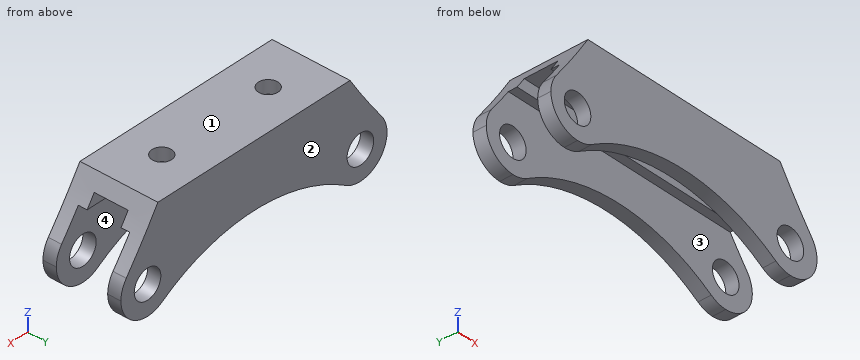
```python
from build123d import *

# Parameters (mm, degrees)
EXTRUDE1_DEPTH            = 47.625
SKETCH4_R                 = 4.7625
SPHERICALHOLES_DEPTH      = 13.7
SPHERICALHOLES_DEPTH_BACK = 13.7
FILLET1_R                 = 9.525
SKETCH5_R                 = 3.175
EXTRUDE2_DEPTH            = 5.318
EXTRUDE3_START            = -47.625
SKETCH6_W                 = 3.81
SKETCH6_H                 = 2.8575
EXTRUDE3_DEPTH            = 95.25
CUT_EXTRUDE1_DEPTH        = 26.4
CUT_EXTRUDE3_DEPTH        = 26.4


with BuildPart() as part:
    # Sketch2 → Extrude1 (new body, symmetric)
    with BuildSketch(Plane(origin=(0, 0, 0), x_dir=(0, 0, -1), z_dir=(1, 0, 0))):
        Polygon((4.318, -8.382), (4.318, 8.382), (31.75, 8.382), (31.75, 12.7), (0, 12.7), (0, -12.7), (31.75, -12.7), (31.75, -8.382), align=None)
    extrude(amount=EXTRUDE1_DEPTH, both=True)

    # Sketch4 → SphericalHoles (cut, two sides)
    with BuildSketch(Plane(origin=(0, 0, 0), x_dir=(1, 0, 0), z_dir=(0, 1, 0))) as sphericalholes_sk:
        with Locations((38.1, 22.225)):
            Circle(SKETCH4_R)
        with Locations((-38.1, 22.225)):
            Circle(SKETCH4_R)
    extrude(amount=SPHERICALHOLES_DEPTH, mode=Mode.SUBTRACT)
    extrude(sphericalholes_sk.sketch, amount=-SPHERICALHOLES_DEPTH_BACK, mode=Mode.SUBTRACT)

    # Fillet1
    fillet1_edges = [part.edges().sort_by_distance(p)[0] for p in [
        (-47.625, 10.541, -31.75),
        (47.625, -10.541, -31.75),
        (47.625, 10.541, -31.75),
        (-47.625, -10.541, -31.75),
    ]]
    fillet(fillet1_edges, radius=FILLET1_R)

    # Sketch5 → Extrude2 (cut, through all)
    with BuildSketch(Plane(origin=(0, 0, -4.318), x_dir=(-1, 0, 0), z_dir=(0, 0, -1))):
        with Locations((19.05, 0)):
            Circle(SKETCH5_R)
        with Locations((-19.05, 0)):
            Circle(SKETCH5_R)
    extrude(amount=-EXTRUDE2_DEPTH, mode=Mode.SUBTRACT)

    # Sketch6 → Extrude3 (add)
    with BuildSketch(Plane(origin=(0, 0, 0), x_dir=(0, 0, -1), z_dir=(1, 0, 0)).offset(EXTRUDE3_START)):
        with Locations((6.223, -6.95325)):
            Rectangle(SKETCH6_W, SKETCH6_H)
        with Locations((6.223, 6.95325)):
            Rectangle(SKETCH6_W, SKETCH6_H)
    extrude(amount=EXTRUDE3_DEPTH)

    # Sketch12 → Cut-Extrude1 (cut, through all)
    with BuildSketch(Plane(origin=(0, 12.7, 0), x_dir=(1, 0, 0), z_dir=(0, 1, 0))):
        with BuildLine():
            Line((-34.3916, 0), (-47.625, 0))
            Line((-47.625, 0), (-47.625, 22.225))
            ThreePointArc((-47.625, 22.225), (-47.136208414, 19.212930529), (-45.72, 16.51))
            ThreePointArc((-45.72, 16.51), (-39.881889157, 8.374329594), (-34.3916, 0))
        make_face()
        with BuildLine():
            Line((47.625, 22.225), (47.625, 0))
            Line((47.625, 0), (34.3916, 0))
            ThreePointArc((34.3916, 0), (39.881889157, 8.374329594), (45.72, 16.51))
            ThreePointArc((45.72, 16.51), (47.136208414, 19.212930529), (47.625, 22.225))
        make_face()
    extrude(amount=-CUT_EXTRUDE1_DEPTH, mode=Mode.SUBTRACT)

    # Sketch13 → Cut-Extrude3 (cut, through all)
    with BuildSketch(Plane(origin=(0, 12.7, 0), x_dir=(1, 0, 0), z_dir=(0, 1, 0))):
        with BuildLine():
            Line((38.1, 31.75), (-38.1, 31.75))
            ThreePointArc((-38.1, 31.75), (-35.390312481, 31.356441209), (-32.904545455, 30.20828736))
            ThreePointArc((-32.904545455, 30.20828736), (0, 20.444107304), (32.904545455, 30.20828736))
            ThreePointArc((32.904545455, 30.20828736), (35.390312481, 31.356441209), (38.1, 31.75))
        make_face()
    extrude(amount=-CUT_EXTRUDE3_DEPTH, mode=Mode.SUBTRACT)


solid = part.part
```
The model under review builds one solid part; all positions refer to its coordinate system, in mm. Face numbers are marked on the shaded views. Give positions to 0.01 mm unless a question says otherwise; leave off trailing zeros. Write each loop counter-clockwise with the first axis right and the second up, starting at its lowest first coordinate (ties: lowest second). Pieces come first, ordered by that corner, then holes. Notation, with made-up numbers: M -38.75,62 L 16.25,62 A21 cw 16.25,84 Z; hole C 26.5,57.25 d7. An arc over 180 degrees is marked long. Write each question's results on one line, items separated by ' | '. Start each with the question number.
1. We need section C-C (z = -19.5). Write out the cut boundary in (x, y), and give its area (3 significant figures).
2. We need section B-B (x = -19.05). Write out the cut boundary in (y, z) (1 decimal).
3. For probe 1 along Y at (x, z) = (3, -18); probe 2 along Y at (x, z) = (-8, -5.5); probe 3 along Z at (x, y) = (-38.1, 11.05), list the stretches that pass through material, from the lowest coordinate up. Write a range as [from, to].
4. We need section A-A (y = 0). Write out the cut boundary in (x, z) (1 decimal), and give its area (3 significant figures).
5. Insertion check: pin 1 Ø5 at (x, y) = (32, -8) entering from -Z; pin 2 Ø10 at (x, y) = (-14, -8.5) entering from -Z; pin 3 Ø8.5 at (x, y) = (-19.05, 0) entering from -Z. Each pin has a flat end and moves straight along its axis. Give the tip position at first contact, or say it passes through.
6. Mouldability with a two-part tool opening along Y and no side actions: class the marked faces 1, 2, 3 and 4 as released by +Y, released by -Y, zero draft, split by the parting line, or undercut.
7. We need section D-D (z = -15). Write out the cut boundary in (x, y).
Results found:
1) outline: M -47.23,-12.7 L -42.01,-12.7 L -42.01,-8.38 L -47.23,-8.38 Z; M -47.23,8.38 L -42.01,8.38 L -42.01,12.7 L -47.23,12.7 Z; M -34.19,-12.7 L 34.19,-12.7 L 34.19,-8.38 L -34.19,-8.38 Z; M -34.19,8.38 L 34.19,8.38 L 34.19,12.7 L -34.19,12.7 Z; M 42.01,-12.7 L 47.23,-12.7 L 47.23,-8.38 L 42.01,-8.38 Z; M 42.01,8.38 L 47.23,8.38 L 47.23,12.7 L 42.01,12.7 Z | area: 681 mm^2
2) outline: M -12.7,-23.5 L -8.4,-23.5 L -8.4,-8.1 L -5.5,-8.1 L -5.5,-4.3 L -3.2,-4.3 L -3.2,0 L -12.7,0 Z; M 3.2,-4.3 L 5.5,-4.3 L 5.5,-8.1 L 8.4,-8.1 L 8.4,-23.5 L 12.7,-23.5 L 12.7,0 L 3.2,0 Z
3) probe 1: y = [-12.7, -8.38], [8.38, 12.7] | probe 2: y = [-12.7, -5.52], [5.52, 12.7] | probe 3: z = [-31.75, -26.99], [-17.46, -5.74]
4) outline: M -37.2,-4.3 L -22.2,-4.3 L -22.2,0 L -34.4,0 A237.7 cw Z; M -15.9,-4.3 L 15.9,-4.3 L 15.9,0 L -15.9,0 Z; M 22.2,-4.3 L 37.2,-4.3 A237.7 cw 34.4,0 L 22.2,0 Z | area: 254 mm^2
5) pin 1: stops at z = -31.03 | pin 2: stops at z = -23.51 | pin 3: stops at z = -4.32
6) face 1: zero draft | face 2: released by +Y | face 3: undercut | face 4: undercut
7) outline: M -44.6,-12.7 L 44.6,-12.7 L 44.6,-8.38 L -44.6,-8.38 Z; M -44.6,8.38 L 44.6,8.38 L 44.6,12.7 L -44.6,12.7 Z
